from build123d import *

# Parameters (mm, degrees)
SKETCH1_W           = 25.4
SKETCH1_H           = 9.525
SKETCH1_R           = 1.5875
BOSS_EXTRUDE1_DEPTH = 1
SKETCH2_R           = 1.5875
BOSS_EXTRUDE2_DEPTH = 6.35
LPATTERN1_COUNT     = 2
LPATTERN1_PITCH     = 19.05


with BuildPart() as part:
    # Sketch1 → Boss-Extrude1 (new body)
    with BuildSketch(Plane(origin=(0, 0, 0), x_dir=(1, 0, 0), z_dir=(0, 1, 0))):
        with Locations((12.7, 4.7625)):
            Rectangle(SKETCH1_W, SKETCH1_H)
        with Locations(Location((4.7625, 4.7625, 0), (0, 0, 270))):
            Circle(SKETCH1_R, mode=Mode.SUBTRACT)
        with Locations(Location((20.6375, 4.7625, 0), (0, 0, 90))):
            Circle(SKETCH1_R, mode=Mode.SUBTRACT)
    extrude(amount=BOSS_EXTRUDE1_DEPTH)

    # Sketch2 → Boss-Extrude2 (add)
    with BuildSketch(Plane.ZY):
        with Locations((0, 1.5875)):
            Circle(SKETCH2_R)
    boss_extrude2 = extrude(amount=-BOSS_EXTRUDE2_DEPTH)

    # LPattern1: Boss-Extrude2 ×2
    with Locations(*[(i * LPATTERN1_PITCH, 0, 0) for i in range(1, LPATTERN1_COUNT)]):
        add(boss_extrude2)


solid = part.part
The model under review builds one solid part; all positions refer to its coordinate system, in mm. A direction names the side the tool comes from. Round coordinates to 2 decimals unless told otherwise and drop trailing zeros. Write each loop counter-clockwise with the first axis right and the second up, starting at its lowest first coordinate (ties: lowest second). Pieces come first, ordered by that corner, then holes. Notation, with made-up numbers: (-2.75, 19.25) - (26.25, 19.25) arc R23 cw to (26.25, 35.25) - close; hole circle Ø11 at (-38.5, 18.25). An arc over 180 degrees is marked (long way). One line per item, written item: value. Start each with the question number.
1. Consider section B-B on y = 1.65. Write out the cut boundary in (x, z).
2. Consider section D-D on y = 0.4. State how many separate pieces and enclosed holes the cut face has, and give its area (3 significant figures).
3. Clearance check with flat-ended pins moving along their axes: P1, Ø1.5, axis at x = 3, z = -2.5, coming from the +Y side; P2, Ø1.5, axis at x = 9.5, y = 1, coming from the +Z side. State where each tip first meets the part, or that it passes through.
4. To check wall thickness, follow L1, parallel to X at y = 1.5, z = -0.75; L2, parallel to X at y = 0.45, z = -4; L3, parallel to Y at x = 10.25, z = -5.5. State the ranges of each line that lie inside material, in increasing order. Write a range as from..to.
5. Machinability: for faces 4 (the face through (12.6, 0.5, 0)), 5 (the face through (19.05, 2, 0)), 6 (the face through (25.4, 0.6, -2.8)), which of the approach directions +Z, -Z, +X, -X, +Y, -Y give a long, thin tool a straight path to every point of the face, cutting with its end or side? Answer none if there is none.
6. The part is to be moulded in two halves that separate along Z. For faces 1 (the face through (5.84, 0.49, -5.93)), 2 (the face through (22.181, 2.869, 0.937)), 3 (the face through (13, 0, -5)), say which applies: released by +Z, released by -Z, zero draft, split by the parting line, or undercut.
7. Consider section A-A on z = 0.25. Write out the cut boundary in (x, y).
8. Consider section C-C on z = -3.75. Write out the cut boundary in (x, y), and give its area (3 significant figures).
Checks:
1. outline: (0, -1.59) - (6.35, -1.59) - (6.35, 1.59) - (0, 1.59) - close; (19.05, -1.59) - (25.4, -1.59) - (25.4, 1.59) - (19.05, 1.59) - close
2. separate pieces: 1
2. enclosed holes: 2
2. area: 239 mm^2
3. P1: stops at y = 1
3. P2: stops at z = 0
4. L1: x = 0..6.35, 19.05..25.4
4. L2: x = 0..3.37, 6.15..19.25, 22.03..25.4
4. L3: y = 0..1
5. face 4: +Z, +Y, -Y
5. face 5: +Z, +Y
5. face 6: +Z, -Z, +X, +Y, -Y
6. face 1: undercut
6. face 2: split by the parting line
6. face 3: zero draft
7. outline: (0, 0.02) - (6.35, 0.02) - (6.35, 3.16) - (0, 3.16) - close; (19.05, 0.02) - (25.4, 0.02) - (25.4, 3.16) - (19.05, 3.16) - close
8. outline: (0, 0) - (3.54, 0) - (3.54, 1) - (0, 1) - close; (5.99, 0) - (19.41, 0) - (19.41, 1) - (5.99, 1) - close; (21.86, 0) - (25.4, 0) - (25.4, 1) - (21.86, 1) - close
8. area: 20.5 mm^2
